```python
from build123d import *

# Parameters (mm, degrees)
SKETCH1_W           = 4
SKETCH1_H           = 4
BOSS_EXTRUDE1_DEPTH = 13.9
SKETCH2_R           = 1.99
BOSS_EXTRUDE2_DEPTH = 4


with BuildPart() as part:
    # Sketch1 → Boss-Extrude1 (new, symmetric)
    with BuildSketch(Plane.XY):
        Rectangle(SKETCH1_W, SKETCH1_H)
    extrude(amount=BOSS_EXTRUDE1_DEPTH, both=True)

    # Sketch2 → Boss-Extrude2 (add)
    with BuildSketch(Plane.XY.offset(13.9)):
        Circle(SKETCH2_R)
    boss_extrude2 = extrude(amount=BOSS_EXTRUDE2_DEPTH)

    # Mirror2: Boss-Extrude2 across plane
    add(boss_extrude2.mirror(Plane.XY))


solid = part.part
```
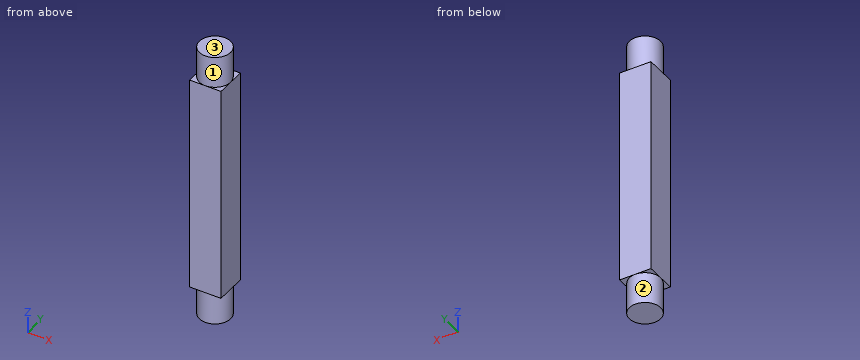
Geometry: final body of the model. Coordinates: model frame, mm. Face numbers are marked on the shaded views. A direction names the side the tool comes from. Give positions to 0.01 mm unless a question says otherwise; leave off trailing zeros. Loops run counter-clockwise (first coordinate to the right, second up) from the corner with the lowest first, then second, coordinate; pieces in that order, holes last. Notation, with made-up numbers: (16, 0.25) - (60, 0.25) arc R14 cw to (60, 21.25) - close; hole circle Ø4 at (21, 60.25). An arc over 180 degrees is marked (long way). Answer as CSV lines item,"result". Start each with the question number.
(1) Section query B-B (x = -1.5). Output: boundary loops of the cut face in (y, z).
(2) Section query A-A (y = 1). Output: boundary loops of the cut face in (x, z).
(3) Reachability of the marked faces 1, 2 and 3 from +Z, -Z, +X, -X, +Y, -Y: full face, straight path, thin tool, end or side. Return the list, or none.
(4) Ray query, line 1 along Z through (x, y) = (1.8, -1.5); line 2 along X through (y, z) = (0.1, -15); line 3 along Y through (x, z) = (1.8, -16). Return the intervals inside material, ascending. Write a range as [from, to].
Worked answers:
1,outline,"(-2, -13.9) - (-1.31, -13.9) - (-1.31, -17.9) - (1.31, -17.9) - (1.31, -13.9) - (2, -13.9) - (2, 13.9) - (1.31, 13.9) - (1.31, 17.9) - (-1.31, 17.9) - (-1.31, 13.9) - (-2, 13.9) - close"
2,outline,"(-2, -13.9) - (-1.72, -13.9) - (-1.72, -17.9) - (1.72, -17.9) - (1.72, -13.9) - (2, -13.9) - (2, 13.9) - (1.72, 13.9) - (1.72, 17.9) - (-1.72, 17.9) - (-1.72, 13.9) - (-2, 13.9) - close"
3,face 1,"+Z"
3,face 2,"-Z"
3,face 3,"+Z, +X, -X, +Y, -Y"
4,line 1,"z = [-13.9, 13.9]"
4,line 2,"x = [-1.99, 1.99]"
4,line 3,"y = [-0.85, 0.85]"
